Check sheet for the modelled part. Datum: model origin and axes. Units: mm. Face numbers are marked on the shaded views. A direction names the side the tool comes from. Give positions to 0.01 mm unless a question says otherwise; leave off trailing zeros. Order: outer loops, then holes, each group sorted by start corner. A loop starts at its lowest first (then second) coordinate and runs counter-clockwise, first axis right, second up.
Item 1: Material ranges on line 1 along Y through (x, z) = (-0.05, 3); line 2 along Z through (x, y) = (2.55, 0.7); line 3 along Y through (x, z) = (0.15, 5), recorded low to high.
Item 2: Sectioned sample at A-A on z = 6.5. Record the boundary of the cut face in (x, y), and give its area (3 significant figures).
Item 3: Sectioned sample at C-C on y = 0.9. Record the boundary of the cut face in (x, z), and give its area (3 significant figures).
Item 4: Access from +Z, -Z, +X, -X, +Y, -Y to the whole of each face (thin tool, end or side, straight path). Record for the marked faces 1 and 2.
Item 5: Sectioned sample at B-B on x = 0.4. Record the boundary of the cut face in (y, z).
Item 6: Gauge pin test, flat ends, axial feed: P1, Ø2, axis at x = -1.5, y = 1, coming from the +Z side; P2, Ø1, axis at x = -2.5, z = 8.5, coming from the -Y side. Record the tip position at first contact, or that the pin passes through.
Item 7: Sectioned sample at D-D on z = -1.5. Record the boundary of the cut face in (x, y), and give its area (3 significant figures).
from build123d import *

# Parameters (mm, degrees)
SKETCH_1_R        = 2.5
EXTRUDE_1_DEPTH   = 5.5
SKETCH_2_R        = 2.9
EXTRUDE_2_DEPTH   = 1
EXTRUDE_1_2_DEPTH = 7


with BuildPart() as part:
    # 草图1 → Extrude 1 (new body)
    with BuildSketch(Plane.XY):
        Circle(SKETCH_1_R)
    extrude(amount=EXTRUDE_1_DEPTH)

    # 草图2 → 拉伸2 (add)
    with BuildSketch(Plane.XY.offset(5.5)):
        Circle(SKETCH_2_R)
    extrude(amount=-EXTRUDE_2_DEPTH)

    # 草图5 → 旋转2 (revolve)
    with BuildSketch(Plane(origin=(0, 0, 0), x_dir=(0, 0, -1), z_dir=(1, 0, 0)), mode=Mode.PRIVATE) as revolve_2_sk:
        with BuildLine():
            Line((0, 2.5), (0, 0))
            Line((0, 0), (2.5, 0))
            ThreePointArc((2.5, 0), (1.767766953, 1.767766953), (0, 2.5))
        make_face()
    revolve(revolve_2_sk.sketch.rotate(Axis((0, 0, -2.5), (0, 0, 1)), 90), axis=Axis((0, 0, -2.5), (0, 0, 1)))

    # 草图6 → Extrude 1 2 (add)
    with BuildSketch(Plane.XY.offset(5.5)):
        with BuildLine():
            ThreePointArc((2.35, 0), (2.6, -0.25), (2.85, 0))
            Line((2.85, 0), (2.35, 0))
        make_face()
        with BuildLine():
            Line((2.35, 0), (2.85, 0))
            ThreePointArc((2.85, 0), (2.6, 0.25), (2.35, 0))
        make_face()
        with BuildLine():
            ThreePointArc((0, -0.25), (0.176776695, -0.176776695), (0.25, 0))
            Line((0.25, 0), (0, 0))
            Line((0, 0), (0, -0.25))
        make_face()
        with BuildLine():
            Line((0, 0), (0.25, 0))
            ThreePointArc((0.25, 0), (0.176776695, 0.176776695), (0, 0.25))
            Line((0, 0.25), (0, 0))
        make_face()
        with BuildLine():
            Line((0, -0.25), (0, 0))
            Line((0, 0), (-0.25, 0))
            ThreePointArc((-0.25, 0), (-0.176776695, -0.176776695), (0, -0.25))
        make_face()
        with BuildLine():
            Line((-0.25, 0), (0, 0))
            Line((0, 0), (0, 0.25))
            ThreePointArc((0, 0.25), (-0.176776695, 0.176776695), (-0.25, 0))
        make_face()
        with BuildLine():
            ThreePointArc((-2.85, 0), (-2.6, -0.25), (-2.35, 0))
            Line((-2.35, 0), (-2.85, 0))
        make_face()
        with BuildLine():
            Line((-2.85, 0), (-2.35, 0))
            ThreePointArc((-2.35, 0), (-2.6, 0.25), (-2.85, 0))
        make_face()
    extrude(amount=EXTRUDE_1_2_DEPTH)


solid = part.part
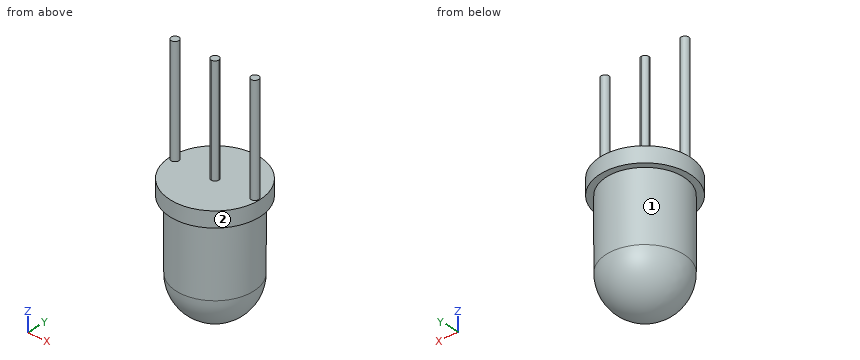
Report:
1. line 1: y = -2.5 to 2.5
1. line 2: z = 4.5 to 5.5
1. line 3: y = -2.9 to 2.9
2. outline: circle Ø0.5 at (-2.6, 0); circle Ø0.5 at (0, 0); circle Ø0.5 at (2.6, 0)
2. area: 0.589 mm2
3. outline: (-2.76, 4.5) - (-2.33, 4.5) - (-2.33, 0) arc R2.33 ccw to (2.33, 0) - (2.33, 4.5) - (2.76, 4.5) - (2.76, 5.5) - (-2.76, 5.5) - close
3. area: 35.1 mm2
4. face 1: -Z
4. face 2: +Z, -Z
5. outline: (-2.87, 4.5) - (-2.47, 4.5) - (-2.47, 0) arc R2.47 ccw to (2.47, 0) - (2.47, 4.5) - (2.87, 4.5) - (2.87, 5.5) - (-2.87, 5.5) - close
6. P1: stops at z = 5.5
6. P2: stops at y = -0.25
7. outline: circle Ø4 at (0, 0)
7. area: 12.6 mm2
